Check sheet for the modelled part. Datum: model origin and axes. Units: mm. A direction names the side the tool comes from. Round coordinates to 2 decimals unless told otherwise and drop trailing zeros. Loops run counter-clockwise (first coordinate to the right, second up) from the corner with the lowest first, then second, coordinate; pieces in that order, holes last. Notation, with made-up numbers: (73.5, 17) -> (96.5, 17) arc R24 cw to (96.5, 34) -> close; hole circle Ø9 at (50, 88.25). An arc over 180 degrees is marked (long way). One line per item, written item: value. Start each with the question number.
1. Cross-section at C-C on y = 25.5. Record the cut outline in (x, z), then the cut area to 3 significant figures.
2. Cross-section at D-D on x = -88. Record the cut outline in (y, z).
3. Go/stop test with flat-tipped pins: pin 1 (1.5 mm diameter, centred on x = -33.5, y = 29.5, fed in from +Z); pin 2 (21.5 mm diameter, centred on x = -92, y = 31.5, fed in from -Z); pin 3 (10 mm diameter, centred on x = -48, y = 29.5, fed in from -Z). Record where each tip stops, or that it passes through.
4. Set-up check for faces 4 (the face through (-50, 25, 7)), 5 (the face through (-40, 5, 9)), 6 (the face through (-13, 25, 12)), 7 (the face through (-12, 25, 15)): record each of +Z, -Z, +X, -X, +Y, -Y from which the full face is reachable in a straight line by a thin tool's end or side.
5. Cross-section at B-B on z = 13. Count the separate pieces of the cut face and the enclosed holes in it, then the cut area to 3 significant figures.
6. Material ranges on L1, parallel to X at y = 39, z = 13.75; L2, parallel to X at y = 16, z = 10.25; L3, parallel to X at y = 19.5, z = 7.75, recorded low to high.
7. Release check for a two-part mould opening along Y. For faces 1 (the face through (-65, 40, 9)), 2 (the face through (-70, 25, 12)), 3 (the face through (-56, 50, 6)) record: +Y half, -Y half, draft (parallel to the pull), parting line (faces both ways), or undercut.
8. Cross-section at A-A on x = -24. Record the cut outline in (y, z), then the cut area to 3 significant figures.
from build123d import *

# Parameters (mm, degrees)
F0_W      = 100
F0_H      = 50
F1_DEPTH  = 15
F2_W      = 10
F2_H      = 10
F3_DEPTH  = 15
F4_R      = 10
F5_R      = 10
F6_W      = 40
F6_H      = 5
F7_DEPTH  = 50
F8_W      = 40
F8_H      = 44
F8_W_2    = 10
F8_H_2    = 10
F8_W_3    = 27
F8_W_4    = 3
F9_DEPTH  = 7
F10_DEPTH = 12


with BuildPart() as f1:
    # F0 (on Top) → F1 (new body)
    with BuildSketch(Plane.XY):
        with Locations((-50, 25)):
            Rectangle(F0_W, F0_H)
    extrude(amount=F1_DEPTH)

    # F2 (on face) → F3 (cut, through all)
    with BuildSketch(Plane.XY.offset(15)):
        with Locations((-20, 40)):
            Rectangle(F2_W, F2_H)
        with Locations((-80, 10)):
            Rectangle(F2_W, F2_H)
        with Locations((-20, 10)):
            Rectangle(F2_W, F2_H)
        with Locations((-20, 25)):
            Rectangle(F2_W, F2_H)
        with Locations((-40, 40)):
            Rectangle(F2_W, F2_H)
        with Locations((-60, 40)):
            Rectangle(F2_W, F2_H)
        with Locations((-60, 10)):
            Rectangle(F2_W, F2_H)
        with Locations((-40, 10)):
            Rectangle(F2_W, F2_H)
        with Locations((-80, 40)):
            Rectangle(F2_W, F2_H)
        with Locations((-80, 25)):
            Rectangle(F2_W, F2_H)
    extrude(amount=-F3_DEPTH, mode=Mode.SUBTRACT)

    # F4
    f4_edges = [f1.edges().sort_by_distance(p)[0] for p in [
        (0, 50, 7.5),
    ]]
    fillet(f4_edges, radius=F4_R)

    # F5
    f5_edges = [f1.edges().sort_by_distance(p)[0] for p in [
        (0, 0, 7.5),
    ]]
    fillet(f5_edges, radius=F5_R)

    # F6 (on face) → F7 (cut, through all)
    with BuildSketch(Plane.XZ):
        with Locations((-50, 12.5)):
            Rectangle(F6_W, F6_H)
    extrude(amount=-F7_DEPTH, mode=Mode.SUBTRACT)

    # F8 (on face) → F9 (cut)
    with BuildSketch(Plane(origin=(0, 0, 0), x_dir=(1, 0, 0), z_dir=(0, 0, -1))):
        with Locations((-50, -25)):
            Rectangle(F8_W, F8_H)
        with Locations((-60, -40)):
            Rectangle(F8_W_2, F8_H_2, mode=Mode.SUBTRACT)
        with Locations((-40, -40)):
            Rectangle(F8_W_2, F8_H_2, mode=Mode.SUBTRACT)
        with Locations((-60, -10)):
            Rectangle(F8_W_2, F8_H_2, mode=Mode.SUBTRACT)
        with Locations((-40, -10)):
            Rectangle(F8_W_2, F8_H_2, mode=Mode.SUBTRACT)
        with Locations((-86.5, -25)):
            Rectangle(F8_W_3, F8_H)
        with Locations((-80, -40)):
            Rectangle(F8_W_2, F8_H_2, mode=Mode.SUBTRACT)
        with Locations((-80, -25)):
            Rectangle(F8_W_2, F8_H_2, mode=Mode.SUBTRACT)
        with Locations((-80, -10)):
            Rectangle(F8_W_2, F8_H_2, mode=Mode.SUBTRACT)
        with BuildLine():
            Line((-27, -3), (-27, -47))
            Line((-27, -47), (-10.2426406871, -47))
            ThreePointArc((-10.2426406871, -47), (-5.1213203436, -44.8786796564), (-3, -39.7573593129))
            Line((-3, -39.7573593129), (-3, -10))
            ThreePointArc((-3, -10), (-5.0502525317, -5.0502525317), (-10, -3))
            Line((-10, -3), (-27, -3))
        make_face()
        with Locations((-20, -40)):
            Rectangle(F8_W_2, F8_H_2, mode=Mode.SUBTRACT)
        with Locations((-20, -25)):
            Rectangle(F8_W_2, F8_H_2, mode=Mode.SUBTRACT)
        with Locations((-20, -10)):
            Rectangle(F8_W_2, F8_H_2, mode=Mode.SUBTRACT)
        with Locations((-28.5, -25)):
            Rectangle(F8_W_4, F8_H)
        with Locations((-71.5, -25)):
            Rectangle(F8_W_4, F8_H)
        with Locations((-20, -40)):
            Rectangle(F8_W_2, F8_H_2)
        with Locations((-80, -25)):
            Rectangle(F8_W_2, F8_H_2)
        with Locations((-80, -10)):
            Rectangle(F8_W_2, F8_H_2)
        with Locations((-20, -25)):
            Rectangle(F8_W_2, F8_H_2)
    extrude(amount=-F9_DEPTH, mode=Mode.SUBTRACT)

    # F8 (on face) → F10 (cut)
    with BuildSketch(Plane(origin=(0, 0, 0), x_dir=(1, 0, 0), z_dir=(0, 0, -1))):
        with Locations((-86.5, -25)):
            Rectangle(F8_W_3, F8_H)
        with Locations((-80, -40)):
            Rectangle(F8_W_2, F8_H_2, mode=Mode.SUBTRACT)
        with Locations((-80, -25)):
            Rectangle(F8_W_2, F8_H_2, mode=Mode.SUBTRACT)
        with Locations((-80, -10)):
            Rectangle(F8_W_2, F8_H_2, mode=Mode.SUBTRACT)
        with BuildLine():
            Line((-27, -3), (-27, -47))
            Line((-27, -47), (-10.2426406871, -47))
            ThreePointArc((-10.2426406871, -47), (-5.1213203436, -44.8786796564), (-3, -39.7573593129))
            Line((-3, -39.7573593129), (-3, -10))
            ThreePointArc((-3, -10), (-5.0502525317, -5.0502525317), (-10, -3))
            Line((-10, -3), (-27, -3))
        make_face()
        with Locations((-20, -40)):
            Rectangle(F8_W_2, F8_H_2, mode=Mode.SUBTRACT)
        with Locations((-20, -25)):
            Rectangle(F8_W_2, F8_H_2, mode=Mode.SUBTRACT)
        with Locations((-20, -10)):
            Rectangle(F8_W_2, F8_H_2, mode=Mode.SUBTRACT)
    extrude(amount=-F10_DEPTH, mode=Mode.SUBTRACT)


solid = f1.part
Taken from the geometry:
1. outline: (-100, 12) -> (-85, 12) -> (-85, 15) -> (-100, 15) -> close; (-75, 12) -> (-73, 12) -> (-73, 7) -> (-27, 7) -> (-27, 12) -> (-25, 12) -> (-25, 15) -> (-30, 15) -> (-30, 10) -> (-70, 10) -> (-70, 15) -> (-75, 15) -> close; (-15, 12) -> (-3, 12) -> (-3, 0) -> (0, 0) -> (0, 15) -> (-15, 15) -> close
1. area: 306 mm2
2. outline: (0, 0) -> (3, 0) -> (3, 12) -> (47, 12) -> (47, 0) -> (50, 0) -> (50, 15) -> (0, 15) -> close
3. pin 1: stops at z = 10
3. pin 2: stops at z = 12
3. pin 3: stops at z = 7
4. face 4: -Z, -X
4. face 5: +Z, -Z
4. face 6: -Z
4. face 7: +Z, +X, -X, +Y, -Y
5. separate pieces: 2
5. enclosed holes: 6
5. area: 2,360 mm2
6. L1: x = -100 to -85, -75 to -70, -30 to -25, -15 to 0
6. L2: x = -73 to -70, -30 to -27, -3 to 0
6. L3: x = -73 to -27, -3 to 0
7. face 1: undercut
7. face 2: draft
7. face 3: +Y half
8. outline: (0, 0) -> (3, 0) -> (3, 12) -> (5, 12) -> (5, 15) -> (0, 15) -> close; (15, 12) -> (20, 12) -> (20, 15) -> (15, 15) -> close; (30, 12) -> (35, 12) -> (35, 15) -> (30, 15) -> close; (45, 12) -> (47, 12) -> (47, 0) -> (50, 0) -> (50, 15) -> (45, 15) -> close
8. area: 132 mm2
